```python
from build123d import *

# Parameters (mm, degrees)
SKETCH1_W               = 136.398
SKETCH1_H               = 309.88
EXTRUDE2_DEPTH          = 160.528
SKETCH3_R               = 50.8
EXTRUDE3_DEPTH          = 62.484
CUT_EXTRUDE1_DEPTH      = 19.05
CUT_EXTRUDE1_DEPTH_BACK = 62.484
SKETCH5_R               = 49.149


with BuildPart() as part:
    # Sketch1 → Extrude2 (new body)
    with BuildSketch(Plane(origin=(0, 0, 0), x_dir=(1, 0, 0), z_dir=(0, 1, 0))):
        with Locations((68.199, 154.94)):
            Rectangle(SKETCH1_W, SKETCH1_H)
    extrude(amount=EXTRUDE2_DEPTH)

    # Sketch3 → Extrude3 (add)
    with BuildSketch(Plane(origin=(0, 160.528, 0), x_dir=(-1, 0, 0), z_dir=(0, 1, 0))):
        with Locations(Location((-68.199, -154.94, 0), (0, 0, 270))):
            Circle(SKETCH3_R)
    extrude(amount=EXTRUDE3_DEPTH)

    # Sketch5 → Cut-Extrude1 (cut, two sides: drawn at the far end of the back side and taken through both)
    with BuildSketch(Plane(origin=(0, 223.012, 0), x_dir=(-1, 0, 0), z_dir=(0, 1, 0)).offset(-CUT_EXTRUDE1_DEPTH_BACK)):
        with Locations(Location((-68.199, -154.94, 0), (0, 0, 90))):
            Circle(SKETCH5_R)
    extrude(amount=CUT_EXTRUDE1_DEPTH + CUT_EXTRUDE1_DEPTH_BACK, mode=Mode.SUBTRACT)


solid = part.part
```
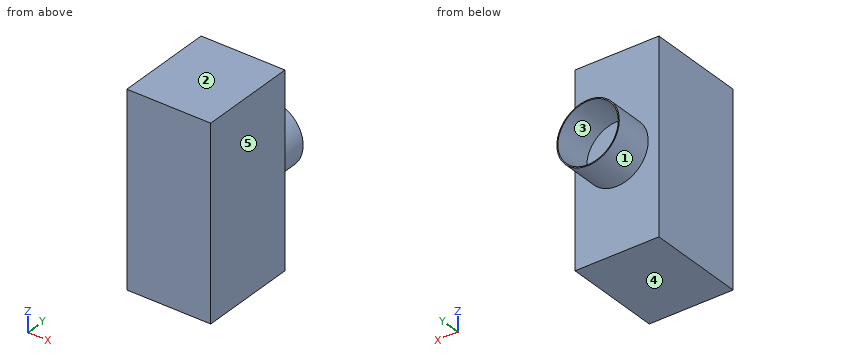
Can you work these out from the model? Positions are in its coordinate system, mm. Face numbers are marked on the shaded views. A direction names the side the tool comes from. Give positions to 0.01 mm unless a question says otherwise; leave off trailing zeros. Write each loop counter-clockwise with the first axis right and the second up, starting at its lowest first coordinate (ties: lowest second). Pieces come first, ordered by that corner, then holes. Notation, with made-up numbers: (31, 84) - (81, 84) arc R9 cw to (81, 98) - close; hole circle Ø5 at (71.25, 59.5). An arc over 180 degrees is marked (long way). Write item = value, one per line. Start each with the question number.
1. Imagine slicing it at B-B (x = 113). Please give me the cut outline in (y, z).
2. On a 3-axis mill with a long thin cutter (end or side, diameter ignored), from which of +Z, -Z, +X, -X, +Y, -Y can I reach the whole of each face in a straight line? I mean the marked faces 1 and 2. Say none if no direction works.
3. Thinking about a two-plate mould opening in X: for the marked faces 3, 4 and 5, which applies, released by +X, released by -X, zero draft, split by the parting line, or undercut?
4. Imagine slicing it at A-A (z = -154.94). Please give me the cut outline in (x, y), and give its area (3 significant figures).
5. Imagine slicing it at D-D (x = 12). Please give me the cut outline in (y, z).
6. Please list where these lines run through material, in increasing order: line 1 (X direction, y = 183, z = -154.94); line 2 (Y direction, x = 85.5, z = -241.5); line 3 (Z direction, x = 34, y = 201.5).
7. For pin 1 (10 mm diameter, centred on x = 30.5, z = -91.5, fed in from +Y); pin 2 (3 mm diameter, centred on y = 174.5, z = -115, fed in from -X); pin 3 (12 mm diameter, centred on x = 68.5, y = 180, fed in from +Z), each with a flat end and sliding along its axis, tell me the tip position at first contact or that it passes through.
8. Imagine slicing it at C-C (y = 165). Please give me the cut outline in (x, z), and give its area (3 significant figures).
Worked answers:
q1.outline = (0, -309.88) - (160.53, -309.88) - (160.53, -178.89) - (223.01, -178.89) - (223.01, -175.15) - (160.53, -175.15) - (160.53, -134.73) - (223.01, -134.73) - (223.01, -130.99) - (160.53, -130.99) - (160.53, 0) - (0, 0) - close
q2.face_1 = +Y
q2.face_2 = +Z, +X, -X, +Y, -Y
q3.face_3 = undercut
q3.face_4 = zero draft
q3.face_5 = released by +X
q4.outline = (0, 0) - (136.4, 0) - (136.4, 160.53) - (119, 160.53) - (119, 223.01) - (117.35, 223.01) - (117.35, 160.53) - (19.05, 160.53) - (19.05, 223.01) - (17.4, 223.01) - (17.4, 160.53) - (0, 160.53) - close
q4.area = 22,100 mm2
q5.outline = (0, -309.88) - (160.53, -309.88) - (160.53, 0) - (0, 0) - close
q6.line_1 = 17.4 to 19.05, 117.35 to 119
q6.line_2 = 0 to 160.53
q6.line_3 = -192.5 to -190.24, -119.64 to -117.38
q7.pin_1 = 160.53
q7.pin_2 = 34.99
q7.pin_3 = -104.14
q8.outline = circle Ø101.6 at (68.2, -154.94); hole circle Ø98.3 at (68.2, -154.94)
q8.area = 518 mm2
